Autodesk Inventor part; units mm, degrees
ref_plane "YZ Plane" through (0, 0, 0) normal (1, 0, 0) x (0, 1, 0)
ref_plane "XZ Plane" through (0, 0, 0) normal (0, 1, 0) x (-1, 0, 0)
ref_plane "XY Plane" through (0, 0, 0) normal (0, 0, 1) x (1, 0, 0)
sketch "Sketch1" plane through (0, 0, 0) normal (0, 0, 1) x (1, 0, 0)
  line L0 (-70, 2) -> (70, 2)
  line L1 (70, 2) -> (70, -2)
  line L2 (70, -2) -> (-70, -2)
  line L3 (-70, -2) -> (-70, 2)
  line L4 (-70, 2) -> (70, -2) construction
  line L5 (70, 2) -> (-70, -2) construction
  line L6 (-70, 2) -> (44.4369, 116.4369)
  line L7 (-70, 2) -> (91.8383, 2) construction
  line L8 (70, 2) -> (-21.2026, 93.2026)
  line L9 (-64.3431, 2) -> (2.8284, 69.1716)
  line L10 (-2.8284, 69.1716) -> (64.3431, 2)
  circle A0 centre (0, 69.1716) radius 3.5
  circle A1 centre (0, 69.1716) radius 5
  circle A2 centre (-67.6199, 0) radius 3.5
  circle A3 centre (-67.6199, 0) radius 5
  circle A4 centre (69.5355, 2.4645) radius 3.5
  circle A5 centre (69.5355, 2.4645) radius 5
  circle A6 centre (29.8984, 39.897) radius 3.5
  circle A7 centre (29.8984, 39.897) radius 5
  line L11 (27.6414, 44.3586) -> (-27.6414, 44.3586)
  line L12 (-27.6414, 44.3586) -> (-27.6414, 52.2202)
  line L13 (-27.6414, 52.2202) -> (-24.6414, 52.2202)
  line L14 (-24.6414, 52.2202) -> (-24.6414, 47.3586)
  line L15 (27.6414, 44.3586) -> (27.6414, 52.2202)
  line L16 (27.6414, 52.2202) -> (24.6414, 52.2202)
  line L17 (24.6414, 52.2202) -> (24.6414, 47.3586)
  circle A8 centre (0, 69.1716) radius 50
  circle A9 centre (0, 69.1716) radius 53
  circle A10 centre (0, 69.1716) radius 57.3
  circle A11 centre (0, 69.1716) radius 60.3
  arc A12 (2.1548, 16.1686) -> (-2.1058, 16.2485) centre (-0.005, 14.6373) ccw
  arc A13 (33.4747, 28.0809) -> (30.3172, 25.699) centre (32.9561, 25.4847) ccw
  line L18 (-2.1058, 16.2485) -> (-2.1315, 16.2145)
  line L19 (-0.1162, 2) -> (-0.1162, -3.5)
  circle A14 centre (-30.1308, 39.897) radius 3.5
  circle A15 centre (-30.1308, 39.897) radius 5
  line L20 (-70.2324, 2) -> (69.7676, -2) construction
  circle A16 centre (-30.1308, 39.897) radius 3.5
  circle A17 centre (-30.1308, 39.897) radius 5
  line L21 (-56, -2) -> (-56, 16)
  line L22 (-52, 20) -> (-52, -2)
  line L23 (-2.1315, 16.2145) -> (-2.1315, 11.9112)
  line L24 (-4.1487, 16.3342) -> (-4.1487, 12.022)
  line L25 (64.3431, 2) -> (64.3431, -2)
  line L26 (66, -2) -> (66, 13.8793)
  line L27 (66, 10) -> (55.978, 16.022)
  line L28 (66, 6) -> (54.3212, 12.022)
  line L29 (64.3431, 2) -> (64.3431, 6.8543)
  point P0 (0, 0)
  point P1 (1.8262, 64.517)
  point P2 (25.0868, 41.2564)
  point P3 (31.2578, 35.0853)
  point P4 (64.3431, 2)
  point P5 (-1.8262, 64.517)
  point P6 (-4.6546, 67.3454)
  point P7 (-67.0344, 4.9656)
  point P8 (-63.0374, -2)
  point P9 (67.2842, -2)
  point P10 (66, 6)
  point P11 (34.36, 37.64)
  point P12 (4.6546, 67.3454)
  point P13 (-41.2009, 25.1423)
  point P14 (41.2009, 25.1423)
  point P15 (39.0783, 27.2648)
  point P16 (-39.0783, 27.2648)
  point P17 (-36.0358, 30.3074)
  point P18 (36.0358, 30.3074)
  point P19 (33.9128, 32.4303)
  point P20 (-33.9128, 32.4303)
  point P21 (2.1218, 16.2141)
  point P22 (-31.3061, 35.0371)
  point P23 (-25.2709, 41.0722)
  point P24 (-27.7217, 44.2783)
  point P25 (-34.5122, 37.4878)
  point P26 (-56, 7)
  point P27 (-52, 2)
  point P28 (-52, 14.3431)
  point P29 (-56, 10.3431)
  point P30 (-56, 2)
  point P31 (44.0293, 27.9707)
  point P32 (41.2009, 113.2009)
  point P33 (1.8262, 73.8262)
  point P34 (0, 66.3431)
  point P35 (0, 72)
  point P36 (21.9846, 44.3586)
  point P37 (63.9523, 2.3909)
  point P38 (-21.9846, 44.3586)
  point P39 (64.5572, 2)
  point P40 (-1.8262, 73.8262)
  point P41 (-44.0293, 27.9707)
  point P42 (70, -1.78)
  point P43 (-26.636, 39.7071)
  point P44 (-29.941, 36.4021)
  point P45 (36.7413, 35.2587)
  point P46 (38.8642, 33.1358)
  point P47 (41.9067, 30.0933)
  point P48 (64.3431, 2)
  dimension "d14" = 10
  dimension "d16" = 10
  dimension "d0" = 140
  dimension "d1" = 4
  dimension "d2" = 45
  dimension "d3" = 4
  dimension "d6" = 4
  dimension "d7" = 4
  dimension "d8" = 4
  dimension "d9" = 7
  dimension "d10" = 10
  dimension "d11" = 7
  dimension "d12" = 10
  dimension "d13" = 7
  dimension "d15" = 7
  dimension "d17" = 3
  dimension "d18" = 3
  dimension "d21" = 3
  dimension "d22" = 3
  dimension "d23" = 4.3
  dimension "d24" = 100
  dimension "d42" = 4
  dimension "d43" = 14
  dimension "d62" = 4
  dimension "d63" = 4
  dimension "d64" = 4
  dimension "d65" = 8
extrude "Extrusion1" add sketch "Sketch1" along normal blind 10 contours L19 L2 L22 L0 | L0 L25 L2 L19 | L29 L28 A5 L0 | L0 A5 L26 L2 L25 | L22 L2 L21 L0 | L0 L21 L9 L22 | A5 L26 L0 | L0 L26 A5 | L10 A11 L8 L28 | L22 L6 A11 L9 | L9 L21 L6 L22 | L8 L27 L26 | A11 L9 A10 L10 | L10 A10 L8 A11 | A11 L6 A10 L9 | L10 A9 L8 A10 | A10 L6 A9 L9 | A9 A13 A12 L18 L9 A8 L10 | L10 A8 L8 A9 | A10 L24 A9 L23 | A9 L6 A8 L9 | L10 A7 L8 A8 | A8 L6 A15 L9 | A7 L10 A6 | L10 A6 L8 A7 | A15 L6 A14 L9 | L9 A14 A15 | A7 L8 A6 L10 | L10 L11 A7 | L8 A6 A7 | A15 L6 A14 | L10 A1 L8 L11 | A14 L6 A15 L9 | L6 L11 L9 A15 | A1 L8 A0 L6 | L6 A0 L8 A1 | A1 L9 A0 L10 | L10 A0 L8 A1 | L11 L6 A1 L9 | L8 A0 L6 A1 | A1 L6 A0 L9
extrude "Extrusion2" cut sketch "Sketch1" along normal blind 10 contours A9 A13 | L18 A12 A9
sketch "Sketch3" plane through (-70, -2, 0) normal (0, -1, 0) x (1, 0, 0)
  line L0 (134.3431, 0) -> (134.3431, 10)
  line L1 (5.6569, 0) -> (5.6569, 10)
  circle A0 centre (23, 5) radius 2.5
  circle A1 centre (128, 5) radius 2.5
  line L2 (140, 0) -> (140, 10)
  line L3 (14, 10) -> (136, 10)
  point P0 (70, 0)
  point P1 (0, 10)
  point P2 (133.7935, 10)
  point P3 (18, 10)
  dimension "d34" = 5
  dimension "d35" = 5
  dimension "d36" = 105
  dimension "d37" = 12
  dimension "d38" = 5
  dimension "d39" = 5
extrude "Extrusion4" cut sketch "Sketch3" against normal up to surface (4 mm away)
sketch "Sketch6" plane through (0, 0, 10) normal (0, 0, 1) x (1, 0, 0)
  line L0 (-0.8413, 73.4692) -> (1.2373, 73.4692)
  line L1 (1.2373, 73.4692) -> (1.2373, 76.4217)
  line L2 (1.2373, 76.4217) -> (-0.8413, 76.4217)
  line L3 (-0.8413, 76.4217) -> (-0.8413, 73.4692)
  point P0 (0, 0)
extrude "Extrusion7" add sketch "Sketch6" against normal blind 3
sketch "Sketch4" plane through (0, 0, 0) normal (0, 0, -1) x (-1, 0, 0)
  circle A0 centre (0, 69.1716) radius 3.5
  arc A1 (-4.6546, 67.3454) -> (-1.8262, 64.517) centre (0, 69.1716) ccw
  line L0 (-0.9508, 73.5061) -> (0.9164, 73.5061)
  line L1 (0.9164, 73.5061) -> (0.9164, 76.8255)
  line L2 (0.9164, 76.8255) -> (-0.9508, 76.8255)
  line L3 (-0.9508, 76.8255) -> (-0.9508, 73.5061)
  point P0 (0, 0)
  point P1 (3.5355, 65.136)
  point P2 (4.6546, 67.3454)
  point P3 (3.5355, 65.636)
  point P4 (3.5355, 65.636)
  point P5 (1.8262, 64.517)
  point P6 (-3.4452, 68.5548)
  point P7 (-0.6168, 65.7263)
extrude "Extrusion5" add sketch "Sketch4" against normal blind 3 contours L3 L2 L1 L0
sketch "Sketch5" plane through (-56, -2, 0) normal (0, -1, 0) x (1, 0, 0)
  circle A0 centre (56.3685, 5) radius 2.5
  circle A1 centre (86.3685, 5) radius 2.5
  line L0 (0, 10) -> (122, 10)
  line L1 (53.8685, 0) -> (53.8685, 10)
  point P0 (56, 0)
  point P1 (119.7935, 10)
  point P2 (-14, 10)
  point P3 (126, 10)
  point P4 (4, 10)
  dimension "d52" = 5
  dimension "d53" = 5
  dimension "d54" = 5
  dimension "d55" = 0
  dimension "d56" = 30
  dimension "d57" = 2.5
extrude "Extrusion6" cut sketch "Sketch5" against normal up to surface (4 mm away)
properties part number "BigCageP2"
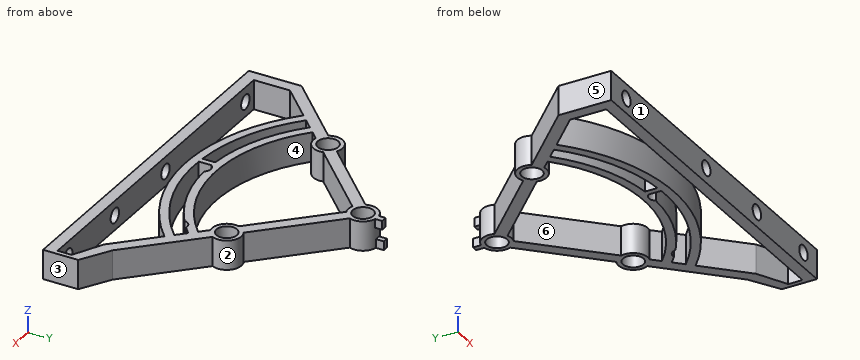
Design review of the part built by this model. Coordinates are the model's own, in mm. Face numbers are marked on the shaded views. A direction names the side the tool comes from. Round coordinates to 2 decimals unless told otherwise and drop trailing zeros. Write each loop counter-clockwise with the first axis right and the second up, starting at its lowest first coordinate (ties: lowest second). Pieces come first, ordered by that corner, then holes.
Item 1: For the marked faces 5 and 6, list the 3-axis set-ups (+Z, -Z, +X, -X, +Y, -Y) from which the entire face can be reached by the end or side of a thin tool; tool diameter is ignored.
Item 2: Consider section C-C on x = -21.5. Give the boundary of the cut face in (y, z).
Item 3: Draft analysis for pull direction Y (two halves, no side actions). For the marked faces 1, 2, 3 and 4, state which applies: released by +Y, released by -Y, zero draft, split by the parting line, or undercut.
Item 4: Wall thickness on L1, parallel to Y at x = 15, z = 6; L2, parallel to Y at x = 22, z = 1; L3, parallel to Z at x = 58, y = 0: over which ranges is each line inside the solid? List them lowest first.
Item 5: For pin 1 Ø6 at (y, z) = (22.5, 4) entering from +X; pin 2 Ø8 at (x, y) = (-19.5, 36) entering from +Z; pin 3 Ø2 at (y, z) = (76, 2) entering from -X; pin 4 Ø4.5 at (x, z) = (30.37, 5) entering from +Y, all flat-tipped, find the tip position at first contact; note any pin that passes through.
Item 6: Consider section D-D on y = 56.5. Give the boundary of the cut face in (x, z).
Item 7: Consider section A-A on y = 4.5. Give the boundary of the cut face in (x, z), and give its area (3 significant figures).
Item 8: Consider section B-B on x = -47. Give the boundary of the cut face in (y, z), and give its area (3 significant figures).
Check values:
1. face 5: +Z, -Z, -X, +Y, -Y
1. face 6: +Z, -Z
2. outline: (-2, 0) - (2, 0) - (2, 10) - (-2, 10) - close; (12.83, 0) - (16.06, 0) - (16.06, 10) - (12.83, 10) - close; (20.73, 0) - (24.03, 0) - (24.03, 10) - (20.73, 10) - close; (44.84, 0) - (50.5, 0) - (50.5, 10) - (44.84, 10) - close
3. face 1: released by -Y
3. face 2: undercut
3. face 3: zero draft
3. face 4: undercut
4. L1: y = -2 to 2, 10.77 to 13.87, 18.34 to 21.47, 51.34 to 57
4. L2: y = -2 to 2, 13.03 to 16.26, 20.95 to 24.27, 44.34 to 50
4. L3: z = 0 to 2.5, 7.5 to 10
5. pin 1: stops at x = 52.5
5. pin 2: passes through
5. pin 3: stops at x = -0.92
5. pin 4: stops at y = 44.9
6. outline: (-15.5, 0) - (-9.84, 0) - (-9.84, 10) - (-15.5, 10) - close; (9.84, 0) - (15.5, 0) - (15.5, 10) - (9.84, 10) - close
7. outline: (-56, 0) - (-52, 0) - (-52, 10) - (-56, 10) - close; (64.34, 0) - (66, 0) - (66, 10) - (64.34, 10) - close
7. area: 56.6 mm2
8. outline: (-2, 0) - (2, 0) - (2, 2.5) - (-2, 2.5) - close; (-2, 7.5) - (2, 7.5) - (2, 10) - (-2, 10) - close; (19.34, 0) - (25, 0) - (25, 10) - (19.34, 10) - close
8. area: 76.6 mm2
